The listing builds one solid part. Answer for the finished solid, in the listing's coordinates (mm). A direction names the side the tool comes from. Give positions to 0.01 mm unless a question says otherwise; leave off trailing zeros. Loops run counter-clockwise (first coordinate to the right, second up) from the corner with the lowest first, then second, coordinate; pieces in that order, holes last. Notation, with made-up numbers: M 12,-10 L 40,-10 A27 ccw 40,24 Z; hole C 76,-25 d3. An arc over 180 degrees is marked long. Use one line per item in the form item = value. Start each with the question number.
1. The part is cut by section B-B (y = -28). Write down the section's boundary in (x, z) (3 decimals).
2. The mould has two halves that part along Y. Classify faces 1 (the face through (-44, 24, 2.6)), 2 (the face through (-58.537, 44.348, 0.789)), 3 (the face through (-57.14, -44.357, 0.789)): released by +Y, released by -Y, zero draft, split by the parting line, or undercut.
3. Straight lines are drawn through the part: line 1 (Y direction, x = -56.75, z = 0.55); line 2 (Z direction, x = 17, y = -30.5); line 3 (Z direction, x = -3.5, y = -8). For each, find the intervals that lie inside material, in ascending order. Write a range as from..to.
4. The part is cut by section A-A (x = 8). Write down the section's boundary in (y, z), and give its area (3 significant figures).
5. The part is cut by section C-C (x = 33). Write down the section's boundary in (y, z).
6. The part is cut by section D-D (z = -1.65). Write down the section's boundary in (x, y) (3 decimals).
7. For faces 4 (the face through (-1, -42, 0)), 5 (the face through (-56, 24, 1.6)), 6 (the face through (-58.498, -44.387, 0.789)), 7 (the face through (-11, 10, 2.6)), 8 (the face through (-1, 41, 0)), determine the directions among +Z, -Z, +X, -X, +Y, -Y from which every point of the face is accessible in a straight line to the end or side of a thin tool.
8. Each of these flat-tipped pins is pushed along its axis until it touches: pin 1 Ø1 at (x, z) = (-26.5, -2) entering from +Y; pin 2 Ø10 at (x, y) = (-29, -26) entering from +Z; pin 3 Ø0.7 at (x, z) = (7.5, 2) entering from -Y. Where does it stop, or does it pass through?
from build123d import *

# Parameters (mm, degrees)
SKETCH1_R           = 1.8
SKETCH1_W           = 98.1
SKETCH1_H           = 2.2
BOSS_EXTRUDE1_DEPTH = 1.6
BOSS_EXTRUDE2_DEPTH = 1
SKETCH4_W           = 14.077668093
SKETCH4_H           = 14.62437365
BOSS_EXTRUDE3_DEPTH = 1
SKETCH5_W           = 20.774811166
SKETCH5_H           = 1.698532112
BOSS_EXTRUDE4_DEPTH = 2
BOSS_EXTRUDE5_DEPTH = 0.1
SKETCH7_W           = 118.5
SKETCH7_H           = 74.2
BOSS_EXTRUDE6_DEPTH = 2.5
SKETCH9_W           = 118.5
SKETCH9_H           = 74.2
SKETCH9_W_2         = 113.57001823
SKETCH9_H_2         = 71.11304095
CUT_EXTRUDE1_DEPTH  = 2
SKETCH10_W          = 51.801411065
SKETCH10_H          = 5.00599424
BOSS_EXTRUDE7_DEPTH = 3


with BuildPart() as part:
    # Sketch1 → Boss-Extrude1 (new body)
    with BuildSketch(Plane.XY):
        with BuildLine():
            Line((-56.75, 45.1), (56.75, 45.1))
            ThreePointArc((56.75, 45.1), (58.517766953, 44.367766953), (59.25, 42.6))
            Line((59.25, 42.6), (59.25, -42.6))
            ThreePointArc((59.25, -42.6), (58.517766953, -44.367766953), (56.75, -45.1))
            Line((56.75, -45.1), (-56.75, -45.1))
            ThreePointArc((-56.75, -45.1), (-58.517766953, -44.367766953), (-59.25, -42.6))
            Line((-59.25, -42.6), (-59.25, 42.6))
            ThreePointArc((-59.25, 42.6), (-58.517766953, 44.367766953), (-56.75, 45.1))
        make_face()
        with Locations((-56.75, 42.6)):
            Circle(SKETCH1_R, mode=Mode.SUBTRACT)
        with Locations((-56.75, -42.6)):
            Circle(SKETCH1_R, mode=Mode.SUBTRACT)
        with Locations((56.75, -42.6)):
            Circle(SKETCH1_R, mode=Mode.SUBTRACT)
        with Locations((56.75, 42.6)):
            Circle(SKETCH1_R, mode=Mode.SUBTRACT)
        with Locations((7.7, -38.2)):
            Rectangle(SKETCH1_W, SKETCH1_H, mode=Mode.SUBTRACT)
    extrude(amount=BOSS_EXTRUDE1_DEPTH)

    # Sketch2 → Boss-Extrude2 (add)
    with BuildSketch(Plane.XY.offset(1.6)):
        with BuildLine():
            Line((-33.280179083, 35.852893933), (-59.25, 35.852893933))
            Line((-59.25, 35.852893933), (-59.25, 33.025293605))
            ThreePointArc((-59.25, 33.025293605), (-52.297040321, 23.771768976), (-59.25, 14.518244348))
            Line((-59.25, 14.518244348), (-59.25, 11.690644019))
            Line((-59.25, 11.690644019), (-33.280179083, 11.690644019))
            Line((-33.280179083, 11.690644019), (-33.280179083, 35.852893933))
        make_face()
    extrude(amount=BOSS_EXTRUDE2_DEPTH)

    # Sketch4 → Boss-Extrude3 (add)
    with BuildSketch(Plane.XY.offset(1.6)):
        with Locations((-11.344165308, 10.250729194)):
            Rectangle(SKETCH4_W, SKETCH4_H)
    extrude(amount=BOSS_EXTRUDE3_DEPTH)

    # Sketch5 → Boss-Extrude4 (add)
    with BuildSketch(Plane.XY):
        with Locations((39.089422326, 22.92250292)):
            Rectangle(SKETCH5_W, SKETCH5_H)
    extrude(amount=BOSS_EXTRUDE4_DEPTH)

    # Sketch6 → Boss-Extrude5 (add)
    with BuildSketch(Plane.XY.offset(1.6)):
        Polygon((30.227507475, 21.978150543), (48.227507475, 21.978150543), (48.227507475, -14.831552551), (52.545445223, -14.831552551), (52.545445223, -37.1), (-37.778090805, -37.1), (-37.778090805, -14.831552551), (30.227507475, -14.831552551), align=None)
    extrude(amount=BOSS_EXTRUDE5_DEPTH)

    # Sketch7 → Boss-Extrude6 (add)
    with BuildSketch(Plane.XY):
        Rectangle(SKETCH7_W, SKETCH7_H)
    extrude(amount=-BOSS_EXTRUDE6_DEPTH)

    # Sketch9 → Cut-Extrude1 (cut)
    with BuildSketch(Plane(origin=(0, 0, -2.5), x_dir=(-1, 0, 0), z_dir=(0, 0, -1))):
        Rectangle(SKETCH9_W, SKETCH9_H)
        Rectangle(SKETCH9_W_2, SKETCH9_H_2, mode=Mode.SUBTRACT)
    extrude(amount=-CUT_EXTRUDE1_DEPTH, mode=Mode.SUBTRACT)

    # Sketch10 → Boss-Extrude7 (add)
    with BuildSketch(Plane.XY):
        with Locations((2.305465736, 40.952943313)):
            Rectangle(SKETCH10_W, SKETCH10_H)
    extrude(amount=BOSS_EXTRUDE7_DEPTH)


solid = part.part
Derived:
q1.outline = M -59.25,-0.5 L -56.785,-0.5 L -56.785,-2.5 L 56.785,-2.5 L 56.785,-0.5 L 59.25,-0.5 L 59.25,1.6 L 52.545,1.6 L 52.545,1.7 L -37.778,1.7 L -37.778,1.6 L -59.25,1.6 Z
q2.face_1 = zero draft
q2.face_2 = released by +Y
q2.face_3 = undercut
q3.line_1 = -45.1..-44.4, -40.8..40.8, 44.4..45.1
q3.line_2 = -2.5..1.7
q3.line_3 = -2.5..1.6
q4.outline = M -45.1,0 L -39.3,0 L -39.3,1.6 L -45.1,1.6 Z; M -37.1,-0.5 L -35.56,-0.5 L -35.56,-2.5 L 35.56,-2.5 L 35.56,-0.5 L 37.1,-0.5 L 37.1,0 L 45.1,0 L 45.1,1.6 L 43.46,1.6 L 43.46,3 L 38.45,3 L 38.45,1.6 L -14.83,1.6 L -14.83,1.7 L -37.1,1.7 Z
q4.area = 329 mm2
q5.outline = M -45.1,0 L -39.3,0 L -39.3,1.6 L -45.1,1.6 Z; M -37.1,-0.5 L -35.56,-0.5 L -35.56,-2.5 L 35.56,-2.5 L 35.56,-0.5 L 37.1,-0.5 L 37.1,0 L 45.1,0 L 45.1,1.6 L 23.77,1.6 L 23.77,2 L 22.07,2 L 22.07,1.6 L 21.98,1.6 L 21.98,1.7 L -37.1,1.7 Z
q6.outline = M -56.785,-35.557 L 56.785,-35.557 L 56.785,35.557 L -56.785,35.557 Z
q7.face_4 = -Z, +X, -X, -Y
q7.face_5 = +Z, -X
q7.face_6 = +Z, -Z, -X, -Y
q7.face_7 = +Z, +X, -X, -Y
q7.face_8 = -Z, +X, -X, +Y
q8.pin_1 = 35.56
q8.pin_2 = 1.7
q8.pin_3 = -37.1
